```python
from build123d import *

# Parameters (mm, degrees)
F1_DEPTH = 3
F2_W     = 7.4
F2_H     = 15
F2_H_2   = 20
F3_DEPTH = 3
F5_DEPTH = 3
F6_R     = 5


with BuildPart() as f1:
    # F0 (on Top) → F1 (new body)
    with BuildSketch(Plane.XY):
        Polygon((36.469397, -45.240614), (39.645866, 4.759386), (-20.354134, 4.759386), (-11.530603, -45.240614), align=None)
    extrude(amount=F1_DEPTH)

    # F2 (on face) → F3 (cut, through all)
    with BuildSketch(Plane.XY.offset(3)):
        with Locations((30.633425, -7.5)):
            Rectangle(F2_W, F2_H)
        with Locations((15.233425, -10)):
            Rectangle(F2_W, F2_H_2)
        with Locations((-0.166575, -10)):
            Rectangle(F2_W, F2_H_2)
        Polygon((-8.364385, 0), (-15.764385, 0), (-11.530603, -25), (-8.364385, -25), align=None)
    extrude(amount=-F3_DEPTH, mode=Mode.SUBTRACT)

    # F4 (on face) → F5 (cut, through all)
    with BuildSketch(Plane.XY.offset(3)):
        Polygon((4.934109, -37.770947), (-10.364607, -30.358168), (-10.056541, -37.751752), (1.70737, -44.430388), align=None)
    extrude(amount=-F5_DEPTH, mode=Mode.SUBTRACT)

    # F6
    f6_edges = [f1.edges().sort_by_distance(p)[0] for p in [
        (-20.354134, 4.759386, 1.5),
        (39.645866, 4.759386, 1.5),
        (36.469397, -45.240614, 1.5),
        (-11.530603, -45.240614, 1.5),
    ]]
    fillet(f6_edges, radius=F6_R)


solid = f1.part
```
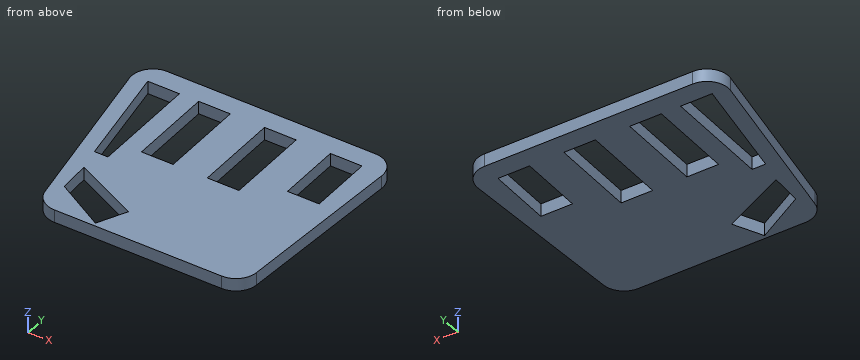
Build history of the part. All positions in model axes, mm. Round coordinates to 2 decimals unless told otherwise and drop trailing zeros. Write each loop counter-clockwise with the first axis right and the second up, starting at its lowest first coordinate (ties: lowest second). Pieces come first, ordered by that corner, then holes.
1) Pin check, flat tips, straight feed: pin 1 (0.9 mm diameter, centred on y = -11.5, z = 1, fed in from +X); pin 2 (0.9 mm diameter, centred on y = -13.5, z = 2, fed in from -X); pin 3 (1.5 mm diameter, centred on y = -5.5, z = 1, fed in from -X). Stop position of each tip, or through.
2) Band-saw the part on C-C, the plane y = -22. List the corners of the cut face in (x, z), and give its area (3 significant figures).
3) Band-saw the part on D-D, the plane x = 2.5. List the corners of the cut face in (y, z), and give its area (3 significant figures).
4) Band-saw the part on A-A, the plane z = 0.5. List the corners of the cut face in (x, y), and give its area (3 significant figures).
5) Drill centre lines: probe 1 along Y at (x, z) = (17, 1.65); probe 2 along Y at (x, z) = (-1, 0.75); probe 3 along X at (y, z) = (-6.5, 1.2). Where is each one in solid material? Low to high.
6) Band-saw the part on B-B, the plane y = -10. List the corners of the cut face in (x, z).
Ans:
1. pin 1: stops at x = 38.64
1. pin 2: stops at x = -17.21
1. pin 3: stops at x = -18.68
2. outline: (-15.63, 0) - (-12.04, 0) - (-12.04, 3) - (-15.63, 3) - close; (-8.36, 0) - (37.95, 0) - (37.95, 3) - (-8.36, 3) - close
2. area: 150 mm2
3. outline: (-45.24, 0) - (-42.79, 0) - (-42.79, 3) - (-45.24, 3) - close; (-36.59, 0) - (-20, 0) - (-20, 3) - (-36.59, 3) - close; (0, 0) - (4.76, 0) - (4.76, 3) - (0, 3) - close
3. area: 71.4 mm2
4. outline: (-19.32, -1.11) - (-12.26, -41.11) arc R5 ccw to (-7.34, -45.24) - (31.78, -45.24) arc R5 ccw to (36.77, -40.56) - (39.31, -0.56) arc R5 ccw to (34.32, 4.76) - (-14.39, 4.76) arc R5 ccw to start; hole (-15.76, 0) - (-11.53, -25) - (-8.36, -25) - (-8.36, 0) - close; hole (-10.36, -30.36) - (-10.06, -37.75) - (1.71, -44.43) - (4.93, -37.77) - close; hole (-3.87, -20) - (3.53, -20) - (3.53, 0) - (-3.87, 0) - close; hole (11.53, -20) - (18.93, -20) - (18.93, 0) - (11.53, 0) - close; hole (26.93, -15) - (34.33, -15) - (34.33, 0) - (26.93, 0) - close
4. area: 2,030 mm2
5. probe 1: y = -45.24 to -20, 0 to 4.76
5. probe 2: y = -45.24 to -42.89, -34.9 to -20, 0 to 4.76
5. probe 3: x = -18.37 to -14.66, -8.36 to -3.87, 3.53 to 11.53, 18.93 to 26.93, 34.33 to 38.93
6. outline: (-17.75, 0) - (-14.07, 0) - (-14.07, 3) - (-17.75, 3) - close; (-8.36, 0) - (-3.87, 0) - (-3.87, 3) - (-8.36, 3) - close; (3.53, 0) - (11.53, 0) - (11.53, 3) - (3.53, 3) - close; (18.93, 0) - (26.93, 0) - (26.93, 3) - (18.93, 3) - close; (34.33, 0) - (38.71, 0) - (38.71, 3) - (34.33, 3) - close
